Could you check a few things on this model? Use its own coordinates, in mm. Face numbers are marked on the shaded views. Round coordinates to 2 decimals unless told otherwise and drop trailing zeros. Write each loop counter-clockwise with the first axis right and the second up, starting at its lowest first coordinate (ties: lowest second). Pieces come first, ordered by that corner, then holes. Notation, with made-up numbers: M 81.25,60 L 136.25,60 A11 ccw 136.25,68 Z; hole C -38.75,76.25 d2. An arc over 180 degrees is marked long. One line per item, written item: value. Start each with the question number.
(1) If I drill on L1, parallel to X at y = 8.5, z = 1.35; L2, parallel to Y at x = -11, z = 1.65; L3, parallel to X at y = 83, z = 4.7, over which ranges is the centre line in solid material (lowest first)?
(2) Thinking about a two-plate mould opening in Z: for the marked faces 1 and 2, which applies, released by +Z, released by -Z, zero draft, split by the parting line, or undercut?
(3) I want a section at C-C on y = 106.5. Please give me the cut outline in (x, z), and give its area (3 significant figures).
(4) I'm going to push a flat-ended pin straight in: pin 1 Ø1.5 at (x, z) = (-35.5, 3) entering from +Y. Where does the tip first touch, or does it pass through?
(5) I want a section at B-B on z = 2.4. Please give me the cut outline in (x, y).
(6) I want a section at A-A on y = 11. Please give me the cut outline in (x, z).
(7) I want a section at D-D on x = -26.5. Please give me the cut outline in (y, z).
Autodesk Inventor part; units mm, degrees
ref_plane "YZ Plane" through (0, 0, 0) normal (1, 0, 0) x (0, 1, 0)
ref_plane "XZ Plane" through (0, 0, 0) normal (0, 1, 0) x (-1, 0, 0)
ref_plane "XY Plane" through (0, 0, 0) normal (0, 0, 1) x (1, 0, 0)
sketch "Sketch1" plane through (0, 0, 0) normal (0, 0, 1) x (1, 0, 0)
  line L0 (-61.8733, -121.208) -> (-61.8733, 128.792)
  line L1 (-61.8733, 128.792) -> (-1.8733, 128.792)
  line L2 (-1.8733, 128.792) -> (-1.8733, -121.208)
  line L3 (-1.8733, -121.208) -> (-61.8733, -121.208)
  line L4 (-66.8733, 113.892) -> (-51.7733, 113.892) construction
  line L5 (-66.8733, 103.792) -> (-1.8733, 103.792) construction
  line L6 (-56.8733, -86.108) -> (-51.7733, -86.108)
  line L7 (-51.7733, -96.208) -> (-56.8733, -96.208)
  line L8 (-51.7733, 13.892) -> (-56.8733, 13.892)
  line L9 (-51.7733, 3.792) -> (-56.8733, 3.792)
  line L10 (-51.7733, 3.792) -> (-51.7733, -86.108) construction
  line L11 (-56.8733, 3.792) -> (-56.8733, -86.108) construction
  line L12 (-51.7733, 13.892) -> (-51.7733, 3.792)
  line L13 (-56.8733, 13.892) -> (-56.8733, 3.792)
  line L14 (-51.7733, 103.792) -> (-51.7733, 13.892) construction
  line L15 (-56.8733, 103.792) -> (-56.8733, 80.792) construction
  line L16 (-51.7733, -86.108) -> (-51.7733, -96.208)
  line L17 (-56.8733, -86.108) -> (-56.8733, -96.208)
  line L18 (-31.8733, 128.792) -> (-31.8733, -121.208) construction
  line L19 (3.1267, 103.792) -> (-61.8733, 103.792) construction
  line L20 (3.1267, 113.892) -> (-61.8733, 113.892) construction
  line L21 (-11.9733, 13.892) -> (-6.8733, 13.892)
  line L22 (-11.9733, 3.792) -> (-6.8733, 3.792)
  line L23 (-11.9733, 13.892) -> (-11.9733, 3.792)
  line L24 (-6.8733, 13.892) -> (-6.8733, 3.792)
  line L25 (-6.8733, -86.108) -> (-6.8733, -96.208)
  line L26 (-6.8733, -86.108) -> (-11.9733, -86.108)
  line L27 (-11.9733, -86.108) -> (-11.9733, -96.208)
  line L28 (-11.9733, -96.208) -> (-6.8733, -96.208)
  line L29 (-1.8733, 128.792) -> (-6.8733, 128.792)
  line L30 (-51.7733, 113.892) -> (-1.8733, 113.892) construction
  line L31 (-61.8733, 128.792) -> (-56.8733, 128.792)
  line L32 (-31.8733, 80.792) -> (-48.3733, 80.792)
  line L33 (-48.3733, 80.792) -> (-48.3733, 128.792)
  line L34 (-31.8733, 80.792) -> (-15.3733, 80.792)
  line L35 (-15.3733, 80.792) -> (-15.3733, 128.792)
  point P0 (0, 0)
  point P1 (-56.8733, 92.292)
  dimension "d6" = 60
  dimension "d7" = 5
  dimension "d11" = 48
  dimension "d12" = 39.8
  dimension "d16" = 25
  dimension "d17" = 16.5
  dimension "d18" = 16.5
extrude "Extrusion1" add sketch "Sketch1" along normal blind 5 contours L0 L1 L33 L32 L34 L35 L2 L3
properties part number "Lifting Sections left"
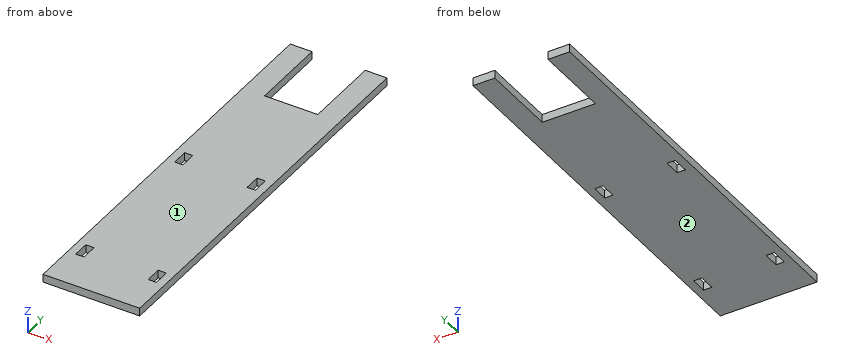
Found:
1. L1: x = -61.87 to -56.87, -51.77 to -11.97, -6.87 to -1.87
1. L2: y = -121.21 to -96.21, -86.11 to 3.79, 13.89 to 128.79
1. L3: x = -61.87 to -48.37, -15.37 to -1.87
2. face 1: released by +Z
2. face 2: released by -Z
3. outline: M -61.87,0 L -48.37,0 L -48.37,5 L -61.87,5 Z; M -15.37,0 L -1.87,0 L -1.87,5 L -15.37,5 Z
3. area: 135 mm²
4. pin 1: stops at y = 80.79
5. outline: M -61.87,-121.21 L -1.87,-121.21 L -1.87,128.79 L -15.37,128.79 L -15.37,80.79 L -48.37,80.79 L -48.37,128.79 L -61.87,128.79 Z; hole M -56.87,-96.21 L -51.77,-96.21 L -51.77,-86.11 L -56.87,-86.11 Z; hole M -56.87,3.79 L -51.77,3.79 L -51.77,13.89 L -56.87,13.89 Z; hole M -11.97,-96.21 L -6.87,-96.21 L -6.87,-86.11 L -11.97,-86.11 Z; hole M -11.97,3.79 L -6.87,3.79 L -6.87,13.89 L -11.97,13.89 Z
6. outline: M -61.87,0 L -56.87,0 L -56.87,5 L -61.87,5 Z; M -51.77,0 L -11.97,0 L -11.97,5 L -51.77,5 Z; M -6.87,0 L -1.87,0 L -1.87,5 L -6.87,5 Z
7. outline: M -121.21,0 L 80.79,0 L 80.79,5 L -121.21,5 Z
